Input: dimensioned drawing with shaded views. Units: mm. Origin: part minimum x, y, z. A direction names the side the tool comes from. Round coordinates to 2 decimals unless told otherwise and drop trailing zeros. Loops run counter-clockwise (first coordinate to the right, second up) from the corner with the lowest first, then second, coordinate; pieces in that order, holes last. Notation, with made-up numbers: M 14,32.25 L 65,32.25 A23 cw 65,59.25 Z; hole C 17.5,12 d2. An arc over 180 degrees is marked long. Put each result on its own line as item: value. Start each with the question number.
1) Reachability of the marked faces 5 and 6 from +Z, -Z, +X, -X, +Y, -Y: full face, straight path, thin tool, end or side. Return the list, or none.
2) Draft query along Z for the marked faces 1, 2, 3 and 4. Return one class per face: +Z half, -Z half, draft (parallel to the pull), parting line (faces both ways), or undercut.
3) Section B-B on y = 0.85. Output: boundary loops of the cut face in (x, z).
4) Pin query (flat end, axial travel): pin 1 (0.8 mm diameter, centred on x = 2, z = 2, fed in from -Y); pin 2 (1.1 mm diameter, centred on x = 3.5, z = 15, fed in from -Y); pin 3 (0.8 mm diameter, centred on x = 2.5, y = 2.5, fed in from +Z). Return the tip coordinate at first contact, or that it passes through.
5) Line query: probe 1 along Z at (x, y) = (8.5, 0.6); probe 2 along X at (y, z) = (0.35, 2.5); probe 3 along X at (y, z) = (1.15, 10.25). Output: solid intervals per line, ascending.
6) Section C-C on z = 17. Output: boundary loops of the cut face in (x, y), plus the area to 3 significant figures.
7) Section A-A on x = 13.5. Output: boundary loops of the cut face in (y, z).
8) Section D-D on x = 3. Output: boundary loops of the cut face in (y, z).
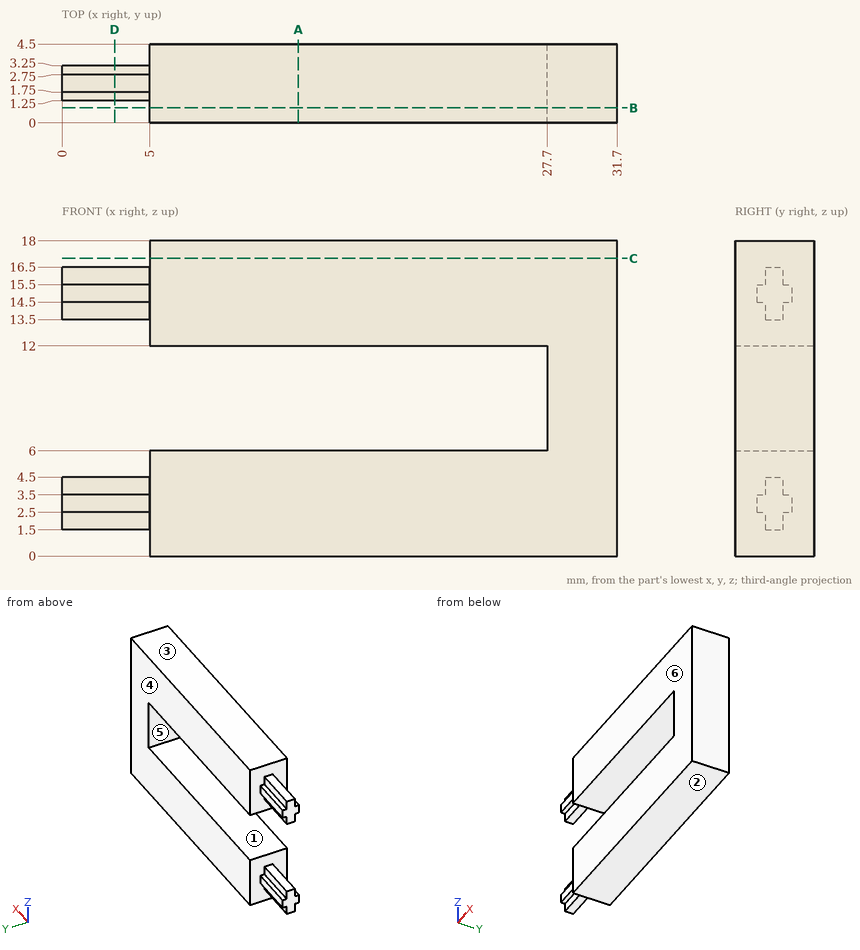
Geometry results:
1. face 5: -X, +Y, -Y
1. face 6: +Z, -Z, +X, -X, -Y
2. face 1: undercut
2. face 2: -Z half
2. face 3: +Z half
2. face 4: draft
3. outline: M 5,0 L 31.7,0 L 31.7,18 L 5,18 L 5,12 L 27.7,12 L 27.7,6 L 5,6 Z
4. pin 1: stops at y = 1.75
4. pin 2: stops at y = 1.25
4. pin 3: stops at z = 16.5
5. probe 1: z = 0 to 6, 12 to 18
5. probe 2: x = 5 to 31.7
5. probe 3: x = 27.7 to 31.7
6. outline: M 5,0 L 31.7,0 L 31.7,4.5 L 5,4.5 Z
6. area: 120 mm²
7. outline: M 0,0 L 4.5,0 L 4.5,6 L 0,6 Z; M 0,12 L 4.5,12 L 4.5,18 L 0,18 Z
8. outline: M 1.25,2.5 L 1.75,2.5 L 1.75,1.5 L 2.75,1.5 L 2.75,2.5 L 3.25,2.5 L 3.25,3.5 L 2.75,3.5 L 2.75,4.5 L 1.75,4.5 L 1.75,3.5 L 1.25,3.5 Z; M 1.25,14.5 L 1.75,14.5 L 1.75,13.5 L 2.75,13.5 L 2.75,14.5 L 3.25,14.5 L 3.25,15.5 L 2.75,15.5 L 2.75,16.5 L 1.75,16.5 L 1.75,15.5 L 1.25,15.5 Z
